Input: part model. Units: mm. Frame: model coordinates. Face numbers are marked on the shaded views. A direction names the side the tool comes from. Round coordinates to 2 decimals unless told otherwise and drop trailing zeros. Loops run counter-clockwise (first coordinate to the right, second up) from the corner with the lowest first, then second, coordinate; pieces in that order, holes last. Notation, with made-up numbers: (68, 40) - (91, 40) arc R15 ccw to (91, 44) - close; hole circle Ø6 at (42.25, -36.75). An arc over 180 degrees is marked (long way). One line per question, with ' | ' between items. Start each with the question number.
from build123d import *

# Parameters (mm, degrees)
F1_DEPTH  = 30
F2_R      = 2
F3_DEPTH  = 25
F4_SIZE   = 1
F5_R      = 2
F6_DEPTH  = 25
F7_SIZE   = 1
F8_R      = 2
F10_DEPTH = 3
F11_SIZE  = 1


with BuildPart() as f1:
    # F0 (on Top) → F1 (new body)
    with BuildSketch(Plane.XY):
        Polygon((-5, 0), (0, 0), (0, 45), (25, 45), (25, 50), (-5, 50), align=None)
    extrude(amount=F1_DEPTH)

    # F2 (on face) → F3 (cut)
    with BuildSketch(Plane.XZ.offset(-45)):
        with Locations((7, 22)):
            Circle(F2_R)
        with Locations((17, 8)):
            Circle(F2_R)
    extrude(amount=-F3_DEPTH, mode=Mode.SUBTRACT)

    # F4
    f4_edges = [f1.edges().sort_by_distance(p)[0] for p in [
        (-2.5, 0, 30),
        (0, 22.5, 30),
        (12.5, 45, 30),
        (25, 47.5, 30),
        (10, 50, 30),
        (-5, 25, 30),
    ]]
    chamfer(f4_edges, length=F4_SIZE)

    # F5 (on face) → F6 (cut)
    with BuildSketch(Plane.YZ):
        with Locations((35, 22)):
            Circle(F5_R)
        with Locations((10, 8)):
            Circle(F5_R)
    extrude(amount=-F6_DEPTH, mode=Mode.SUBTRACT)

    # F7
    f7_edges = [f1.edges().sort_by_distance(p)[0] for p in [
        (0, 0, 14.5),
        (-5, 0, 14.5),
        (25, 45, 14.5),
        (25, 50, 14.5),
        (-5, 50, 14.5),
    ]]
    chamfer(f7_edges, length=F7_SIZE)

    # F8
    f8_edges = [f1.edges().sort_by_distance(p)[0] for p in [
        (0, 45, 14.5),
    ]]
    fillet(f8_edges, radius=F8_R)

    # F9 (on face) → F10 (join)
    with BuildSketch(Plane(origin=(0, 0, 0), x_dir=(1, 0, 0), z_dir=(0, 0, -1))):
        Polygon((20, -45), (0, -25), (0, -45), align=None)
    extrude(amount=-F10_DEPTH)

    # F11
    f11_edges = [f1.edges().sort_by_distance(p)[0] for p in [
        (10, 35, 3),
    ]]
    chamfer(f11_edges, length=F11_SIZE)


solid = f1.part
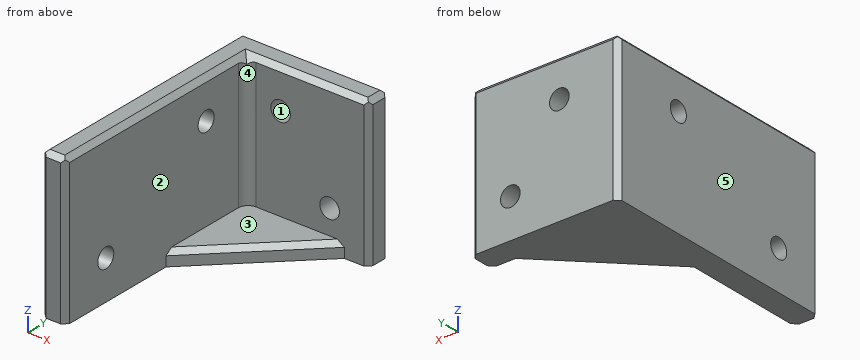
(1) Pin query (flat end, axial travel): P1, Ø5.5, axis at x = 5, y = 38, coming from the +Z side; P2, Ø10, axis at y = 21.5, z = 25.5, coming from the +X side; P3, Ø6.5, axis at x = 17, z = 8, coming from the -Y side. Return the tip coordinate at first contact, or that it passes through.
(2) Section C-C, the plane y = 36. Output: boundary loops of the cut face in (x, z).
(3) Section A-A, the plane x = -2.75. Output: boundary loops of the cut face in (y, z).
(4) Reachability of the marked faces 4 and 5 from +Z, -Z, +X, -X, +Y, -Y: full face, straight path, thin tool, end or side. Return the list, or none.
(5) Section B-B, the plane z = 22. Output: boundary loops of the cut face in (x, y), plus the area to 3 significant figures.
(6) Pull-direction query (Z, two-part tool) for the marked faces 1, 2 and 3; classes: released by +Z, released by -Z, zero draft, split by the parting line, or undercut.
(7) Section D-D, the plane x = 7. Output: boundary loops of the cut face in (y, z).
(8) Line query: line 1 along Z through (x, y) = (-3.9, 10); line 2 along Z through (x, y) = (-3.45, 35); line 3 along Y through (x, z) = (19.5, 11). Output: solid intervals per line, ascending. Write a range as from..to.
Derived:
1) P1: stops at z = 3 | P2: stops at x = 0 | P3: stops at y = 45
2) outline: (-5, 0) - (11, 0) - (11, 2) - (9.59, 3) - (0, 3) - (0, 20.27) - (-5, 20.27) - close; (-5, 23.73) - (0, 23.73) - (0, 29) - (-1, 30) - (-4, 30) - (-5, 29) - close
3) outline: (0, 0) - (50, 0) - (50, 29) - (49, 30) - (1, 30) - (0, 29) - close; hole circle Ø4 at (10, 8); hole circle Ø4 at (35, 22)
4) face 4: +Z, +X, -Y | face 5: +Z, -Z, -X, +Y, -Y
5) outline: (-5, 1) - (-4, 0) - (-1, 0) - (0, 1) - (0, 33) - (-5, 33) - close; (-5, 37) - (0, 37) - (0, 43) arc R2 cw to (2, 45) - (5, 45) - (5, 50) - (-4, 50) - (-5, 49) - close; (9, 45) - (24, 45) - (25, 46) - (25, 49) - (24, 50) - (9, 50) - close | area: 333 mm²
6) face 1: undercut | face 2: zero draft | face 3: released by +Z
7) outline: (32, 0) - (50, 0) - (50, 20) - (45, 20) - (45, 3) - (33.41, 3) - (32, 2) - close; (45, 24) - (50, 24) - (50, 29) - (49, 30) - (46, 30) - (45, 29) - close
8) line 1: z = 0..6, 10..30 | line 2: z = 0..20, 24..30 | line 3: y = 45..50
